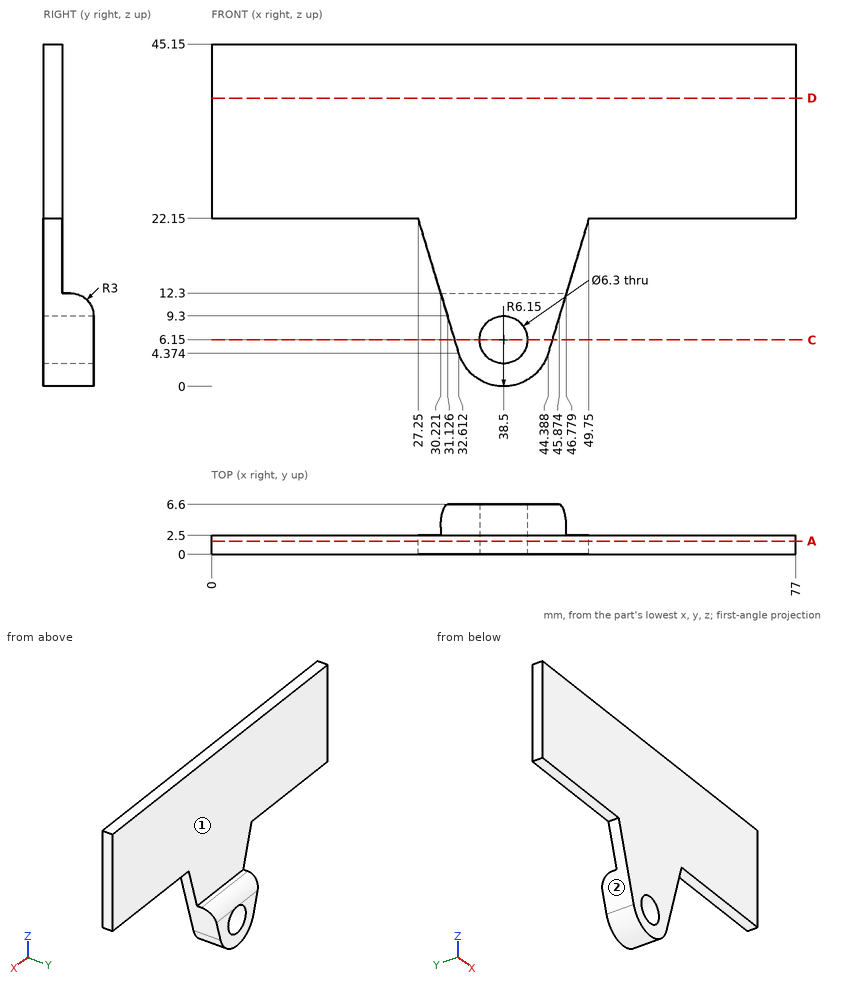
Study the drawing (mm; zero at the part's minimum x, y, z) and answer. A direction names the side the tool comes from. Give positions to 0.01 mm unless a question says otherwise; leave off trailing zeros. Order: outer loops, then holes, each group sorted by start corner. A loop starts at its lowest first (then second) coordinate and runs counter-clockwise, first axis right, second up. Notation, with made-up numbers: M 85,65 L 107,65 A22 ccw 107,83 Z; hole C 13,-20.5 d6. An arc over 180 degrees is marked long. Put each result on its own line as item: value. Start each with the question number.
Item 1: The part is cut by section C-C, the plane z = 6.15. Determine the outline of the cut face in (x, y), and give its area (3 significant figures).
Item 2: Which of the six approach directions +Z, -Z, +X, -X, +Y, -Y give full straight-line access (tool end or side, diameter ignored) to the marked faces 1 and 2?
Item 3: The part is cut by section D-D, the plane z = 38. Determine the outline of the cut face in (x, y).
Item 4: Find the intervals of material crossed by line 1 along Z through (x, y) = (63, 1.75); line 2 along Y through (x, z) = (29.5, 33); line 3 along X through (y, z) = (0.5, 10) (1 decimal), in increasing order.
Item 5: The part is cut by section A-A, the plane y = 1.75. Determine the outline of the cut face in (x, z).
Item 6: Flat-ended cylindrical pins translate along their axes: P1, Ø0.6, axis at x = 37, y = 3, coming from the +Z side; P2, Ø5, axis at x = 51.5, z = 37, coming from the +Y side; P3, Ø2, axis at y = 5, z = 24.5, coming from the +X side; P4, Ø7, axis at x = 38.5, z = 6.15, coming from the -Y side. Find the tip coordinate at first contact, or state that the pin passes through.
Answer key:
1. outline: M 32.08,0 L 35.35,0 L 35.35,6.6 L 32.08,6.6 Z; M 41.65,0 L 44.92,0 L 44.92,6.6 L 41.65,6.6 Z
1. area: 43.2 mm²
2. face 1: +Z, +X, -X, +Y
2. face 2: -Z, -X, +Y, -Y
3. outline: M 0,0 L 77,0 L 77,2.5 L 0,2.5 Z
4. line 1: z = 22.15 to 45.15
4. line 2: y = 0 to 2.5
4. line 3: x = 30.9 to 46.1
5. outline: M 0,22.15 L 27.25,22.15 L 32.61,4.37 A6.15 ccw 44.39,4.37 L 49.75,22.15 L 77,22.15 L 77,45.15 L 0,45.15 Z; hole C 38.5,6.15 d6.3
6. P1: stops at z = 12.3
6. P2: stops at y = 2.5
6. P3: passes through
6. P4: stops at y = 0
